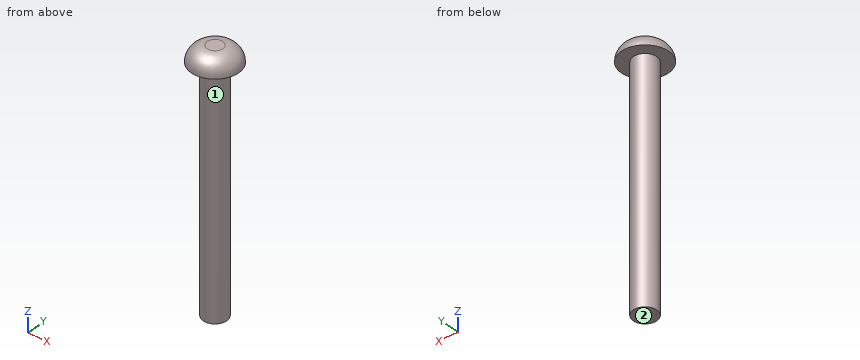
Autodesk Inventor part; units mm, degrees
ref_plane "YZ Plane" through (0, 0, 0) normal (1, 0, 0) x (0, 1, 0)
ref_plane "XZ Plane" through (0, 0, 0) normal (0, 1, 0) x (-1, 0, 0)
ref_plane "XY Plane" through (0, 0, 0) normal (0, 0, 1) x (1, 0, 0)
sketch "スケッチ1" plane through (0, 0, 0) normal (0, 0, 1) x (1, 0, 0)
  circle A0 centre (0, 0) radius 1.5
  dimension "d0" = 3
extrude "押し出し1" add sketch "スケッチ1" along normal blind 30
sketch "スケッチ2" plane through (0, 0, 30) normal (0, 0, 1) x (1, 0, 0)
  circle A0 centre (0, 0) radius 1.5
  circle A1 centre (0, 0) radius 3
  dimension "d3" = 6
extrude "押し出し2" add sketch "スケッチ2" along normal blind 2 contours A0 | A1
fillet "フィレット1" radius 2 1 edges at (-3, 0, 32)
properties part number "M3ボタンボルト15" material "鋼、高強度、低合金"
Can you work these out from the model? Positions are in its coordinate system, mm. Face numbers are marked on the shaded views. A direction names the side the tool comes from. Give positions to 0.01 mm unless a question says otherwise; leave off trailing zeros. Loops run counter-clockwise (first coordinate to the right, second up) from the corner with the lowest first, then second, coordinate; pieces in that order, holes last. Notation, with made-up numbers: (37, 86) - (90, 86) arc R25 ccw to (90, 124) - close; hole circle Ø2 at (8.5, 33). An arc over 180 degrees is marked (long way). Return JSON: item names as keys, results as strings.
1. For the marked faces 1 and 2, which set-ups out of +Z, -Z, +X, -X, +Y, -Y let a thin tool reach every point of the face, with its end or its side?
Output values:
{"face 1": "-Z", "face 2": "-Z, +X, -X, +Y, -Y"}
2. I'm going to push a flat-ended pin straight in: pin 1 Ø1.5 at (x, z) = (1, 14.5) entering from -Y. Where does the tip first touch, or does it pass through?
Output values:
{"pin 1": "stops at y = -1.48"}
3. If I drill on line 1 (Y direction, x = 0, z = 9); line 2 (Z direction, x = -2, y = 0.75); line 3 (Z direction, x = -1.25, y = -2), over which ranges is the centre line in solid material (lowest first)?
Output values:
{"line 1": "y = -1.5 to 1.5", "line 2": "z = 30 to 31.65", "line 3": "z = 30 to 31.47"}
4. I want a section at A-A on z = 21.5. Please give me the cut outline in (x, y), and give its area (3 significant figures).
Output values:
{"outline": "circle Ø3 at (0, 0)", "area": "7.07 mm²"}
